The model under review builds one solid part; all positions refer to its coordinate system, in mm. Give positions to 0.01 mm unless a question says otherwise; leave off trailing zeros. Write each loop counter-clockwise with the first axis right and the second up, starting at its lowest first coordinate (ties: lowest second). Pieces come first, ordered by that corner, then holes. Notation, with made-up numbers: M 75,8.25 L 120,8.25 A16 cw 120,15.25 Z; hole C -2,14.25 d6. An arc over 180 degrees is marked long. Write item = value, one per line. Start each with the question number.
```python
from build123d import *

# Parameters (mm, degrees)
SKETCH1_R           = 15.6845
SKETCH1_R_2         = 2.2479
BOSS_EXTRUDE1_DEPTH = 1.5875
SKETCH2_R           = 15.6845
SKETCH2_R_2         = 12.7
BOSS_EXTRUDE2_DEPTH = 1.5875


with BuildPart() as part:
    # Sketch1 → Boss-Extrude1 (new body)
    with BuildSketch(Plane(origin=(0, 0, 0), x_dir=(1, 0, 0), z_dir=(0, 1, 0))):
        with BuildLine():
            Line((-22.929181133, 3.78943243), (-13.6271, 13.311823526))
            ThreePointArc((-13.6271, 13.311823526), (0, 19.05), (13.6271, 13.311823526))
            Line((13.6271, 13.311823526), (22.929181133, 3.78943243))
            ThreePointArc((22.929181133, 3.78943243), (24.4729, 0), (22.929181133, -3.78943243))
            Line((22.929181133, -3.78943243), (13.6271, -13.311823526))
            ThreePointArc((13.6271, -13.311823526), (0, -19.05), (-13.6271, -13.311823526))
            Line((-13.6271, -13.311823526), (-22.929181133, -3.78943243))
            ThreePointArc((-22.929181133, -3.78943243), (-24.4729, 0), (-22.929181133, 3.78943243))
        make_face()
        with Locations(Location((0, 0, 0), (0, 0, 270))):
            Circle(SKETCH1_R, mode=Mode.SUBTRACT)
        with Locations(Location((-19.05, 0, 0), (0, 0, 270))):
            Circle(SKETCH1_R_2, mode=Mode.SUBTRACT)
        with Locations(Location((19.05, 0, 0), (0, 0, 270))):
            Circle(SKETCH1_R_2, mode=Mode.SUBTRACT)
    extrude(amount=BOSS_EXTRUDE1_DEPTH)

    # Sketch2 → Boss-Extrude2 (add)
    with BuildSketch(Plane.XZ):
        Circle(SKETCH2_R)
        with Locations(Location((0, 0, 0), (0, 0, 270))):
            Circle(SKETCH2_R_2, mode=Mode.SUBTRACT)
    extrude(amount=-BOSS_EXTRUDE2_DEPTH)


solid = part.part
```
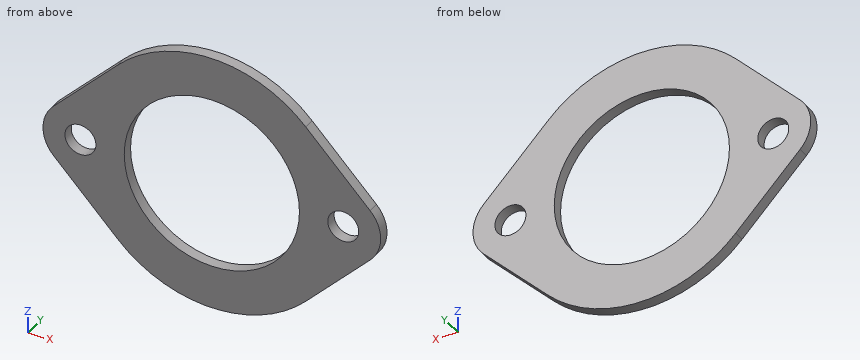
Item 1: To check wall thickness, follow probe 1 along X at (y, z) = (0.55, 0); probe 2 along X at (y, z) = (0.6, 1); probe 3 along Z at (x, y) = (11, 1.2). State the ranges of each line that lie inside material, in increasing order. Write a range as [from, to].
Item 2: We need section C-C, the plane z = 0. Write out the cut boundary in (x, y), and give its area (3 significant figures).
Item 3: Clearance check with a flat-ended pin moving along its axis: P1, Ø2, axis at x = -5.5, z = -10.5, coming from the +Y side. State where the tip first meets the part, or that it passes through.
Item 4: We need section D-D, the plane z = 8. Write out the cut boundary in (x, y).
Item 5: We need section A-A, the plane x = 0. Write out the cut boundary in (y, z).
Item 6: We need section B-B, the plane y = 0.7. Write out the cut boundary in (x, z), and give its area (3 significant figures).
Worked out:
q1.probe_1 = [-24.47, -21.3], [-16.8, -12.7], [12.7, 16.8], [21.3, 24.47]
q1.probe_2 = [-24.38, -21.06], [-17.04, -12.66], [12.66, 17.04], [21.06, 24.38]
q1.probe_3 = [-15.55, -6.35], [6.35, 15.55]
q2.outline = M -24.47,0 L -21.3,0 L -21.3,1.59 L -24.47,1.59 Z; M -16.8,0 L -12.7,0 L -12.7,1.59 L -16.8,1.59 Z; M 12.7,0 L 16.8,0 L 16.8,1.59 L 12.7,1.59 Z; M 21.3,0 L 24.47,0 L 24.47,1.59 L 21.3,1.59 Z
q2.area = 23.1 mm²
q3.P1 = 1.59
q4.outline = M -18.82,0 L -9.86,0 L -9.86,1.59 L -18.82,1.59 Z; M 9.86,0 L 18.82,0 L 18.82,1.59 L 9.86,1.59 Z
q5.outline = M 0,-19.05 L 1.59,-19.05 L 1.59,-12.7 L 0,-12.7 Z; M 0,12.7 L 1.59,12.7 L 1.59,19.05 L 0,19.05 Z
q6.outline = M -22.93,-3.79 L -13.63,-13.31 A19.05 ccw 13.63,-13.31 L 22.93,-3.79 A5.42 ccw 22.93,3.79 L 13.63,13.31 A19.05 ccw -13.63,13.31 L -22.93,3.79 A5.42 ccw Z; hole C -19.05,0 d4.5; hole C 0,0 d25.4; hole C 19.05,0 d4.5
q6.area = 737 mm²
